Autodesk Inventor part; units mm, degrees
ref_plane "Slot Start Plane" through (0, 0, -1.7245) normal (0, 0, 1) x (1, 0, 0)
ref_plane "YZ Plane" through (0, 0, 0) normal (1, 0, 0) x (0, 1, 0)
ref_plane "XZ Plane" through (0, 0, 0) normal (0, 1, 0) x (-1, 0, 0)
ref_plane "Slot Start Plane" through (0, 0, -1.7245) normal (0, 0, 1) x (1, 0, 0)
sketch "Key Profile" plane through (0, 0, 0) normal (1, 0, 0) x (0, 1, 0)
  line L0 (-2, 2.8563) -> (0.684, 1.8794)
  arc A0 (1.6188, -1.1745) -> (0.684, 1.8794) centre (0, 0) ccw
  line L1 (-2, 1.3132) -> (0.1881, 0.5168)
  arc A1 (0, -0.55) -> (0.1881, 0.5168) centre (0, 0) ccw
  line L2 (-2, 2.8563) -> (-2, -0.55)
  line L3 (0, 0) -> (-2, 0) construction
  line L4 (0, -0.55) -> (-2, -0.55)
  line L5 (1.6188, -1.1745) -> (-0.097, -0.55)
  line L6 (6, -5.55) -> (6, 87.7952)
  line L7 (-2, 87.9773) -> (-2, 2.8563)
  arc A2 (6, 87.7952) -> (-2, 87.9773) centre (0, 0) ccw
  line L8 (-2, -0.55) -> (-2, -7.55)
  arc A3 (4, -7.55) -> (6, -5.55) centre (4, -5.55) ccw
  line L9 (-2, -7.55) -> (4, -7.55)
  arc A4 (6, 55.1747) -> (-2, 55.464) centre (0, 0) ccw
  arc A5 (-2, 2.8563) -> (-2, 83.2148) centre (-539.3737, 43.0355) ccw
  point P0 (-0.5, 43.0355)
  point P1 (-0.6441, 55.4963)
  dimension "my_hingeCutRad" = 0.55
  dimension "my_hingeDepth" = 2
  dimension "my_hingeRegCutRad" = 2
  dimension "keyLength" = 88
  dimension "my_KeyHeight" = 8
  dimension "d107" = 20
  dimension "d122" = 4
  dimension "slotOffset" = 1.1745
  dimension "my_backWidth" = 7
  dimension "d128" = 55.5
  dimension "d135" = 1.5
  dimension "d136" = 4.7625
extrude "Upper (u)" add sketch "Key Profile" along normal blind 6.6071 and the other way blind 6.7 contours A5 A4 L6 A3 L9 L8 L4 L5 A0 L0 | L0 A0 L5 L4 A1 L1 L2
extrude "Lower (d)" add sketch "Key Profile" along normal blind 6.6071 and the other way blind 13.4643 contours A5 L7 A2 L6 A4
extrude "Protrusion Cutout" cut sketch "Key Profile" along normal mid plane 4.5 contours L0 A0 L5 L4 A1 L1 L2
fillet "Front Fillet" radius 1.5 1 edges at (-3.4286, 6, 87.7952)
sketch "Slot Sketch" plane through (0, 0, -1.7245) normal (0, 0, 1) x (1, 0, 0)
  line L0 (2.15, -2) -> (2.15, 1)
  line L1 (3.1, 4) -> (-3.1, 4)
  line L2 (-2.15, 1) -> (-2.15, -2)
  line L3 (-2.15, -2) -> (2.15, -2)
  line L4 (0, -2) -> (0, 4) construction
  line L5 (-3.1, 4) -> (-3.1, 1)
  line L6 (-3.1, 1) -> (-2.15, 1)
  line L7 (2.15, 1) -> (3.1, 1)
  line L8 (3.1, 1) -> (3.1, 4)
  point P0 (0, 0)
  dimension "d109" = 2
  dimension "my_slotHeadOffset" = 1
  dimension "my_slotHeadHeight" = 3
  dimension "my_slotHeadWidth" = 6.2
  dimension "my_neckSlotWidth" = 4.3
extrude "Slot" cut sketch "Slot Sketch" against normal through all
fillet "Edge Softening" radius 0.7 13 edges at (6.6071, 5.4142, -6.9642) (6.6071, 1, -7.55) (6.6071, 6, 40.4164) (-6.7, 5.4142, -6.9642) (-6.7, 1, -7.55) (-6.7, 6, 24.8124) (-13.4643, 5.5879, 87.4156) (-13.4643, 1.2899, 87.9905) (-13.4643, 6, 70.7788) (6.6071, 5.5879, 87.4156) (6.6071, 1.2899, 87.9905) (-13.4643, 2.6828, 55.4351) (-10.0821, 6, 55.1747)
equation "\"my_headHeight\" = 3"
equation "\"my_headOffset\" = 1"
equation "\"whiteKeyWidth\" = 20.07143"
properties part number "EKey0"
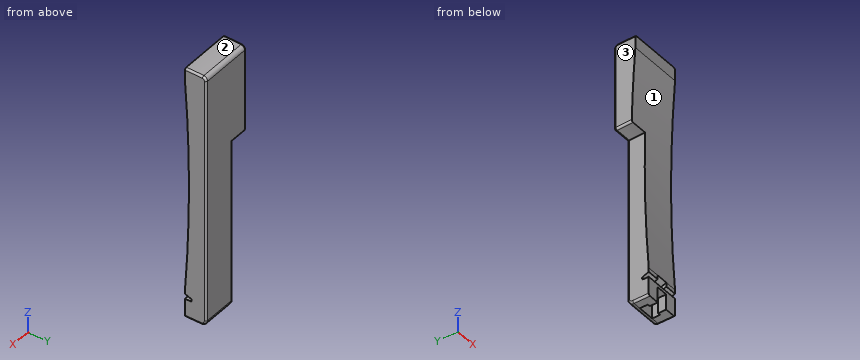
Can you work these out from the model? Positions are in its coordinate system, mm. Face numbers are marked on the shaded views. Give positions to 0.01 mm unless a question says otherwise; leave off trailing zeros. Loops run counter-clockwise (first coordinate to the right, second up) from the corner with the lowest first, then second, coordinate; pieces in that order, holes last. Notation, with made-up numbers: M 39.5,-38 L 49.5,-38 A24 ccw 49.5,-4 Z; hole C -8,48 d10. An arc over 180 degrees is marked long. One line per question, with ' | ' between items. Start each with the question number.
Q1. If we section it at D-D (z = 14): Please give me the cut outline in (x, y), plus the area to 3 significant figures.
Q2. If we mould it in two halves opening along Z, with no side actions, what happens to the marked faces 1, 2 and 3? For each: +Z half, -Z half, draft (parallel to the pull), parting line (faces both ways), or undercut.
Q3. If we section it at A-A (x = -1.25): Please give me the cut outline in (y, z), plus the area to 3 significant figures.
Q4. If we section it at B-B (z = 50): Please give me the cut outline in (x, y) (3 decimals).
Q5. For pin 1 Ø2.5 at (y, z) = (2, -6) entering from -X; pin 2 Ø1 at (x, y) = (-8.5, 3) entering from +Z, each with a flat end and sliding along its axis, tell me the tip position at first contact or that it passes through.
Q6. If we section it at C-C (x = 5): Please give me the cut outline in (y, z), plus the area to 3 significant figures.
Q7. If I drill on line 1 (Z direction, x = 1.75, y = 2.25); line 2 (X direction, y = -0.75, z = 1); line 3 (Z direction, x = 1.5, y = 1.25), over which ranges is the centre line in solid material (lowest first)? Write a range as from..to.
Computed:
1) outline: M -6.7,-1.28 L 6.61,-1.28 L 6.61,5.3 A0.7 ccw 5.91,6 L -6,6 A0.7 ccw -6.7,5.3 Z | area: 96.7 mm²
2) face 1: undercut | face 2: +Z half | face 3: draft
3) outline: M -2,-1.72 L 4,-1.72 L 4,-7.55 A2 ccw 6,-5.55 L 6,86.38 A1.5 ccw 4.58,87.88 A88.02 ccw -2,87.98 L -2,83.21 A538.88 cw -2,2.86 L 0.68,1.88 A2 cw 1.62,-1.17 L -0.1,-0.55 L -2,-0.55 Z | area: 636 mm²
4) outline: M -6.7,-0.545 L 6.607,-0.545 L 6.607,5.3 A0.7 ccw 5.907,6 L -6,6 A0.7 ccw -6.7,5.3 Z
5) pin 1: stops at x = -6.7 | pin 2: stops at z = 87.96
6) outline: M -2,-7.55 L 4,-7.55 A2 ccw 6,-5.55 L 6,86.38 A1.5 ccw 4.58,87.88 A88.02 ccw -2,87.98 L -2,83.21 A538.88 cw -2,2.86 L -2,1.31 L 0.19,0.52 A0.55 cw 0,-0.55 L -2,-0.55 Z | area: 679 mm²
7) line 1: z = -1.72..87.97 | line 2: x = -6.7..-2.25, 2.25..6.61 | line 3: z = -1.72..-1.04, 1.56..87.99
